Autodesk Inventor part; units mm, degrees
ref_plane "YZ Plane" through (0, 0, 0) normal (1, 0, 0) x (0, 1, 0)
ref_plane "XZ Plane" through (0, 0, 0) normal (0, 1, 0) x (-1, 0, 0)
ref_plane "XY Plane" through (0, 0, 0) normal (0, 0, 1) x (1, 0, 0)
sketch "Sketch1" plane through (0, 0, 0) normal (0, 1, 0) x (-1, 0, 0)
  line L0 (0, -6) -> (0, 0)
  line L1 (0, 0) -> (-12, 0)
  line L2 (-12, 0) -> (-12, 13)
  line L3 (-12, 13) -> (0, 13)
  line L4 (0, 13) -> (0, 67)
  line L5 (0, 67) -> (-8, 75)
  line L6 (-8, 75) -> (-67, 75)
  line L7 (-67, 75) -> (-75, 67)
  line L8 (0, -6) -> (-100, -50)
  line L9 (-100, -50) -> (-124.5, -50)
  line L10 (-124.5, -50) -> (-124.5, 0)
  line L11 (-124.5, 0) -> (-118.5, 0)
  line L12 (-118.5, 0) -> (-118.5, 13)
  line L13 (-118.5, 13) -> (-124.5, 13)
  line L14 (-124.5, 13) -> (-124.5, 19)
  line L15 (-124.5, 19) -> (-75, 19)
  line L16 (-75, 19) -> (-75, 67)
  circle A0 centre (-26, 55) radius 4
  circle A1 centre (-49, 55) radius 2.5
  line L17 (-106, -50) -> (-112.5, -50) construction
  line L18 (-112.5, -50) -> (-112.5, 13) construction
  line L19 (-112.5, 13) -> (-106, 13) construction
  line L20 (-106, 13) -> (-106, -50) construction
  dimension "d0" = 13
  dimension "d1" = 12
  dimension "d2" = 6
  dimension "d3" = 6
  dimension "d4" = 6
  dimension "d6" = 75
  dimension "d7" = 8
  dimension "d8" = 5
  dimension "d9" = 23
  dimension "d10" = 106.5
  dimension "d11" = 45
  dimension "d12" = 8
  dimension "d13" = 6.5
  dimension "d14" = 6
  dimension "d15" = 6
  dimension "d16" = 42
  dimension "d17" = 20
  dimension "d18" = 50
  dimension "d19" = 26
extrude "Extrusion1" add sketch "Sketch1" along normal blind 6.5
sketch "Sketch3" plane through (0, 6.5, 0) normal (0, 1, 0) x (1, 0, 0)
  line L0 (124.5, 0) -> (124.5, 50)
  line L1 (124.5, 50) -> (100, 50)
  line L2 (106, 50) -> (112.5, 50)
  line L3 (112.5, 50) -> (112.5, 44)
  line L4 (112.5, 44) -> (106, 44)
  line L5 (106, 44) -> (106, 50)
  dimension "d27" = 6
  dimension "d28" = 6.5
  dimension "d29" = 12
extrude "Extrusion3" cut sketch "Sketch3" against normal through all
chamfer "Chamfer1" distance 2 angle 45 3 edges at (75, 3.25, 19) (124.5, 3.25, 19) (124.5, 3.25, -50)
sketch "Sketch4" plane through (0, 6.5, 0) normal (0, 1, 0) x (1, 0, 0)
  line L0 (124.5, 0) -> (124.5, 48)
  circle A0 centre (26, -55) radius 4
  circle A1 centre (49, -55) radius 2.5
  circle A2 centre (37.5, -47.5) radius 2.25
  circle A3 centre (37.5, -62.5) radius 2.25
  line L1 (37.5, -47.5) -> (37.5, -62.5) construction
  line L2 (26, -55) -> (49, -55) construction
  point P0 (37.5, -55)
  dimension "d35" = 15
  dimension "d36" = 4.5
extrude "Extrusion4" cut sketch "Sketch4" against normal through all contours A2 | A3
sketch "Sketch5" plane through (0, 6.5, 0) normal (0, 1, 0) x (1, 0, 0)
  line L0 (106, 44) -> (106, 50)
  line L1 (100, 50) -> (0, 6)
  line L2 (0, 6) -> (0, 0)
  line L3 (0, 0) -> (12, 0)
  line L4 (12, -13) -> (0, -13)
  line L5 (0, -13) -> (0, -67)
  line L6 (53, 88) -> (6.5, -55) construction
  line L7 (10.7922, 10.7486) -> (32.0112, 76.0025)
  line L8 (32.0112, 76.0025) -> (62.9182, 65.9523)
  line L9 (62.9182, 65.9523) -> (50.6734, 28.2963)
  line L10 (50.6734, 28.2963) -> (10.7922, 10.7486)
  circle A0 centre (6.5, -55) radius 0.9 construction
  circle A1 centre (53, 88) radius 0.9 construction
  point P0 (47.4647, 70.9774)
  dimension "d39" = 42
  dimension "d40" = 6.5
  dimension "d41" = 106
  dimension "d42" = 53
  dimension "d43" = 88
  dimension "d44" = 32.5
  dimension "d45" = 1.8
  dimension "d46" = 17.9
extrude "Extrusion5" add sketch "Sketch5" against normal blind 6.5
sketch "Sketch6" plane through (0, 6.5, 0) normal (0, 1, 0) x (1, 0, 0)
  line L0 (50.6734, 28.2963) -> (62.9182, 65.9523)
  line L1 (62.9182, 65.9523) -> (32.0112, 76.0025)
  line L2 (32.0112, 76.0025) -> (10.7922, 10.7486)
  line L3 (33.6272, 71.2708) -> (39.8086, 69.2608)
  line L4 (39.8086, 69.2608) -> (37.3347, 61.6529)
  line L5 (37.3347, 61.6529) -> (31.1533, 63.6629)
  line L6 (31.1533, 63.6629) -> (33.6272, 71.2708)
  line L7 (52.6469, 65.0861) -> (58.8283, 63.076)
  line L8 (58.8283, 63.076) -> (56.3544, 55.4682)
  line L9 (56.3544, 55.4682) -> (50.173, 57.4782)
  line L10 (50.173, 57.4782) -> (52.6469, 65.0861)
  line L11 (17.2376, 20.8686) -> (23.419, 18.8586)
  line L12 (23.419, 18.8586) -> (20.9451, 11.2507)
  line L13 (20.9451, 11.2507) -> (14.7637, 13.2607)
  line L14 (14.7637, 13.2607) -> (17.2376, 20.8686)
  line L15 (24.8156, -20.5026) -> (30.997, -22.5126)
  line L16 (30.997, -22.5126) -> (28.5231, -30.1205)
  line L17 (28.5231, -30.1205) -> (22.3417, -28.1105)
  line L18 (22.3417, -28.1105) -> (24.8156, -20.5026)
  line L19 (24.9685, 44.6432) -> (31.15, 42.6332)
  line L20 (31.15, 42.6332) -> (28.6761, 35.0253)
  line L21 (28.6761, 35.0253) -> (22.4947, 37.0353)
  line L22 (22.4947, 37.0353) -> (24.9685, 44.6432)
  line L23 (37.185, 17.5368) -> (43.3665, 15.5268)
  line L24 (43.3665, 15.5268) -> (40.8926, 7.9189)
  line L25 (40.8926, 7.9189) -> (34.7112, 9.9289)
  line L26 (34.7112, 9.9289) -> (37.185, 17.5368)
  dimension "d49" = 6.5
  dimension "d50" = 3
  dimension "d52" = 3
  dimension "d53" = 4
  dimension "d54" = 8
  dimension "d57" = 45
  dimension "d58" = 20
  dimension "d59" = 82
  dimension "d60" = 42
extrude "Extrusion6" cut sketch "Sketch6" against normal through all
sketch "Sketch7" plane through (0, 6.5, 0) normal (0, 1, 0) x (1, 0, 0)
  line L0 (32.0112, 76.0025) -> (10.7922, 10.7486)
  line L1 (12, -13) -> (0, -13)
  line L2 (0, -13) -> (0, -67)
  line L3 (5.2631, -58.8039) -> (7.7369, -51.1961) construction
  line L4 (2.8856, -58.0308) -> (5.3595, -50.423)
  line L5 (10.1144, -51.9692) -> (7.6405, -59.577)
  arc A0 (2.8856, -58.0308) -> (7.6405, -59.577) centre (5.2631, -58.8039) ccw
  arc A1 (10.1144, -51.9692) -> (5.3595, -50.423) centre (7.7369, -51.1961) ccw
  point P0 (6.5, -55)
  point P1 (6.5, -55)
  dimension "d63" = 42
  dimension "d64" = 6.5
  dimension "d65" = 5
  dimension "d66" = 8
extrude "Extrusion7" cut sketch "Sketch7" against normal through all
chamfer "Chamfer2" distance 2 angle 45 3 edges at (32.0112, 3.25, -76.0025) (62.9182, 3.25, -65.9523) (50.6734, 3.25, -28.2963)
sketch "Sketch8" plane through (0, 6.5, 0) normal (0, 1, 0) x (1, 0, 0)
  line L0 (12, 0) -> (12, -13)
  line L1 (0, -13) -> (0, -67)
  circle A0 centre (22.217, -6.5) radius 2.25
  point P0 (12, -6.5)
  dimension "d72" = 4.5
  dimension "d73" = 22.217
extrude "Extrusion8" cut sketch "Sketch8" against normal through all
sketch "Sketch9" plane through (0, 6.5, 0) normal (0, 1, 0) x (1, 0, 0)
  line L0 (0, 6) -> (0, 0)
  line L1 (0, 0) -> (12, 0)
  line L2 (34.828, 57.5) -> (41.328, 57.5)
  line L3 (41.328, 57.5) -> (41.328, 49.5)
  line L4 (41.328, 49.5) -> (34.828, 49.5)
  line L5 (34.828, 49.5) -> (34.828, 57.5)
  line L6 (34.828, 34.5) -> (41.328, 34.5)
  line L7 (41.328, 34.5) -> (41.328, 26.5)
  line L8 (41.328, 26.5) -> (34.828, 26.5)
  line L9 (34.828, 26.5) -> (34.828, 34.5)
  circle A0 centre (38.078, 42) radius 2.25
  point P0 (38.078, 49.5)
  dimension "d76" = 8
  dimension "d77" = 6.5
  dimension "d78" = 15
  dimension "d79" = 4.5
  dimension "d80" = 7.5
  dimension "d81" = 38.078
  dimension "d82" = 42
extrude "Extrusion9" cut sketch "Sketch9" against normal through all
sketch "Sketch10" plane through (0, 6.5, 0) normal (0, 1, 0) x (1, 0, 0)
  circle A0 centre (22.217, -6.5) radius 2.25
  line L0 (118.5, -13) -> (118.5, 0)
  line L1 (118.5, 0) -> (124.5, 0)
  line L2 (112.5, 44) -> (106, 44)
  circle A1 centre (93.5, -6.5) radius 2.25
  circle A2 centre (109.25, 28) radius 2.25
  point P0 (109.25, 44)
  dimension "d85" = 25
  dimension "d86" = 28
extrude "Extrusion10" cut sketch "Sketch10" against normal through all contours A1 | A2
equation "\"d2\" = d3"
equation "\"d4\" = d3"
equation "\"d42\" = 0.5 * d41"
properties part number "z_axis_top" material "Plywood, Finish"
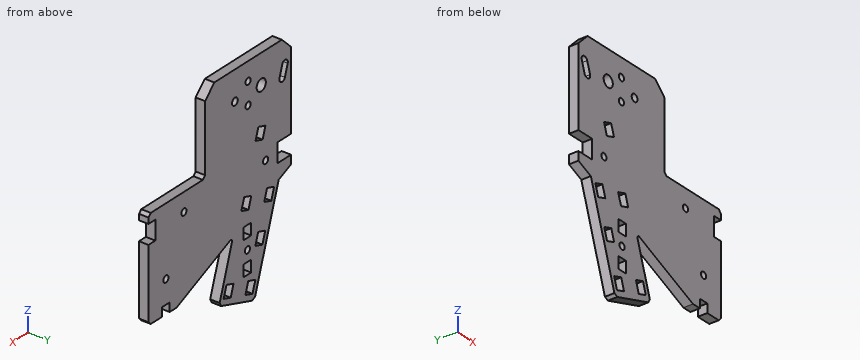
Could you check a few things on this model? Use its own coordinates, in mm. Round coordinates to 2 decimals unless told otherwise and drop trailing zeros. Loops run counter-clockwise (first coordinate to the right, second up) from the corner with the lowest first, then second, coordinate; pieces in that order, holes last. Notation, with made-up numbers: (-9, -35) - (19, -35) arc R15 cw to (19, -25) - close; hole circle Ø4 at (-2.75, -19.5). An arc over 180 degrees is marked (long way). Write item = value, one per line.
1) I'm going to push flat-ended pins straight in: P1, Ø3, axis at x = 39, y = 5, coming from the -Z side; P2, Ø2, axis at y = 5, z = 38.5, coming from the -X side; P3, Ø1.8, axis at x = 121, y = 2.5, coming from the -Z side. Where does each tip first touch, or does it pass through?
Computed:
P1 = -74.22
P2 = 0
P3 = -50
2) Imagine slicing it at D-D (x = 93.5). Please give me the cut outline in (y, z), and give its area (3 significant figures).
Computed:
outline = (0, -47.14) - (6.5, -47.14) - (6.5, 4.25) - (0, 4.25) - close; (0, 8.75) - (6.5, 8.75) - (6.5, 19) - (0, 19) - close
area = 401 mm2
3) Imagine slicing it at C-C (z = 55). Please give me the cut outline in (x, y), and give its area (3 significant figures).
Computed:
outline = (0, 0) - (3.87, 0) - (3.87, 6.5) - (0, 6.5) - close; (9.13, 0) - (22, 0) - (22, 6.5) - (9.13, 6.5) - close; (30, 0) - (46.5, 0) - (46.5, 6.5) - (30, 6.5) - close; (51.5, 0) - (75, 0) - (75, 6.5) - (51.5, 6.5) - close
area = 369 mm2
4) I need wall thicknesses on line 1 along X through (y, z) = (5, 6.5); line 2 along X through (y, z) = (4, 62.5); line 3 along Z through (x, y) = (7, 1.5). Which ranges of each line are inside material? Lowest first, please. Write a range as from..to.
Computed:
line_1 = 12..19.97, 24.47..91.25, 95.75..118.5
line_2 = 0..35.25, 39.75..75
line_3 = -9.08..0, 13..48.81, 60.6..74
5) Imagine slicing it at A-A (x = 109.25). Please give me the cut outline in (y, z), and give its area (3 significant figures).
Computed:
outline = (0, -44) - (6.5, -44) - (6.5, -30.25) - (0, -30.25) - close; (0, -25.75) - (6.5, -25.75) - (6.5, 19) - (0, 19) - close
area = 380 mm2
6) Imagine slicing it at B-B (z = -32.5). Please give me the cut outline in (x, y), and give its area (3 significant figures).
Computed:
outline = (17.87, 0) - (34.83, 0) - (34.83, 6.5) - (17.87, 6.5) - close; (41.33, 0) - (52.04, 0) - (52.04, 6.5) - (41.33, 6.5) - close; (60.23, 0) - (124.5, 0) - (124.5, 6.5) - (60.23, 6.5) - close
area = 598 mm2
